Model file for the job. Use its own axes, mm. A direction names the side the tool comes from. Give positions to 0.01 mm unless a question says otherwise; leave off trailing zeros. Loops run counter-clockwise (first coordinate to the right, second up) from the corner with the lowest first, then second, coordinate; pieces in that order, holes last. Notation, with made-up numbers: M 61.5,4.25 L 67.5,4.25 A24 cw 67.5,30.25 Z; hole C 37.5,64.5 d6. An arc over 180 degrees is marked long. Answer in a Markdown table with one row per item.
```python
from build123d import *

# Parameters (mm, degrees)
F0_R     = 10.5
F0_R_2   = 8.6
F1_DEPTH = 7
F3_W     = 5
F3_H     = 5
F4_DEPTH = 4
F5_W     = 5
F5_H     = 3
F6_DEPTH = 6
F8_DEPTH = 25


with BuildPart() as f1:
    # F0 (on Front) → F1 (new body)
    with BuildSketch(Plane.XZ):
        Circle(F0_R)
        Circle(F0_R_2, mode=Mode.SUBTRACT)
    extrude(amount=F1_DEPTH)

    # F3 (on offset) → F4 (join)
    with BuildSketch(Plane.XY.offset(9)):
        with Locations((0, -3.5)):
            Rectangle(F3_W, F3_H)
    extrude(amount=F4_DEPTH)

    # F5 (on face) → F6 (join)
    with BuildSketch(Plane.YZ.offset(2.5)):
        with Locations((-3.5, 11)):
            Rectangle(F5_W, F5_H)
    extrude(amount=F6_DEPTH)

    # F7 (on face) → F8 (cut)
    with BuildSketch(Plane.XZ.offset(6)):
        Polygon((8.5, 9.5), (8.5, 12.5), (7.633975, 11), align=None)
    extrude(amount=-F8_DEPTH, mode=Mode.SUBTRACT)

    # F9: F1 across plane


with BuildPart() as f1_1:
    add(f1.part)
    add(f1.part.mirror(Plane.YZ))


solid = f1_1.part
```
(1) Flat gauge pins, fed straight in: P1, Ø2, axis at x = -7.5, y = -3, coming from the +Z side; P2, Ø1.2, axis at x = -7, y = -2.5, coming from the -Z side; P3, Ø1, axis at y = -2, z = 2, coming from the -X side. Where does each tip first touch, or does it go through?
Established:
| item | result |
|---|---|
| P1 | stops at z = 12.5 |
| P2 | stops at z = -8.32 |
| P3 | stops at x = -10.39 |
(2) Wall check: L1, parallel to Z at x = 0, y = -3.25; L2, parallel to X at y = -2.25, z = 0; L3, parallel to X at y = -0.25, z = -4.75. Give the ranges that are in metal, low to high.
Established:
| item | result |
|---|---|
| L1 | z = -10.5 to -8.6, 8.6 to 13 |
| L2 | x = -10.5 to -8.6, 8.6 to 10.5 |
| L3 | x = -9.36 to -7.17, 7.17 to 9.36 |
(3) Saw through at B-B, the plane z = 0. Give the cut face in (x, y).
Established:
| item | result |
|---|---|
| outline | M -10.5,-7 L -8.6,-7 L -8.6,0 L -10.5,0 Z; M 8.6,-7 L 10.5,-7 L 10.5,0 L 8.6,0 Z |
(4) Which spindle directions (+Z, -Z, +X, -X, +Y, -Y) get a long thin tool onto all of the face, cutting with end or side? Do faces 1 (the flat face through (-8.073, -3.535, 11.76)), 2 (the flat face through (-5, -4, 12.5)), 3 (the flat face through (5, -4, 12.5)), 4 (the flat face through (0, -1, 11)). Say none if no direction does.
Established:
| item | result |
|---|---|
| face 1 | -X, +Y, -Y |
| face 2 | +Z, -X, +Y, -Y |
| face 3 | +Z, +X, +Y, -Y |
| face 4 | +Z, +Y |
(5) Saw through at C-C, the plane x = 0. Give the cut face in (y, z).
Established:
| item | result |
|---|---|
| outline | M -7,-10.5 L 0,-10.5 L 0,-8.6 L -7,-8.6 Z; M -7,8.6 L 0,8.6 L 0,10.5 L -1,10.5 L -1,13 L -6,13 L -6,10.5 L -7,10.5 Z |
(6) Saw through at D-D, the plane x = -5.25. Give the cut face in (y, z), and give its area (3 significant figures).
Established:
| item | result |
|---|---|
| outline | M -7,-9.09 L 0,-9.09 L 0,-6.81 L -7,-6.81 Z; M -7,6.81 L 0,6.81 L 0,9.09 L -7,9.09 Z; M -6,9.5 L -1,9.5 L -1,12.5 L -6,12.5 Z |
| area | 46.9 mm2 |
(7) Mould opens along Z. For faces 5 (the flat face through (0, -6, 11)), 6 (the flat face through (0, -3, 13)), 7 (the flat face through (8.06, -3.54, 10.26)) say: pulls with the +Z half, pulls with the -Z half, needs draft (parallel to the pull), parting line crosses it, or undercut.
Established:
| item | result |
|---|---|
| face 5 | needs draft |
| face 6 | pulls with the +Z half |
| face 7 | undercut |
(8) Saw through at A-A, the plane y = -3.75. Give the cut face in (x, z), and give its area (3 significant figures).
Established:
| item | result |
|---|---|
| outline | M -8.5,9.5 L -4.47,9.5 A10.5 ccw long 4.47,9.5 L 8.5,9.5 L 7.63,11 L 8.5,12.5 L 2.5,12.5 L 2.5,13 L -2.5,13 L -2.5,12.5 L -8.5,12.5 L -7.63,11 Z; hole C 0,0 d17.2 |
| area | 159 mm2 |
